Source: three-view drawing plus pictorial views. Frame: mm from the lowest corner of the part. A direction names the side the tool comes from. Coordinates: 2 decimals unless noted, no trailing zeros. Write each loop counter-clockwise with the first axis right and the second up, starting at its lowest first coordinate (ties: lowest second). Pieces come first, ordered by that corner, then holes. Notation, with made-up numbers: (12.5, 25) -> (49.5, 25) arc R20 ccw to (49.5, 47) -> close; hole circle Ø2 at (36, 60). An arc over 180 degrees is marked (long way). One line per question, with ' | ' between items. Start each with the question number.
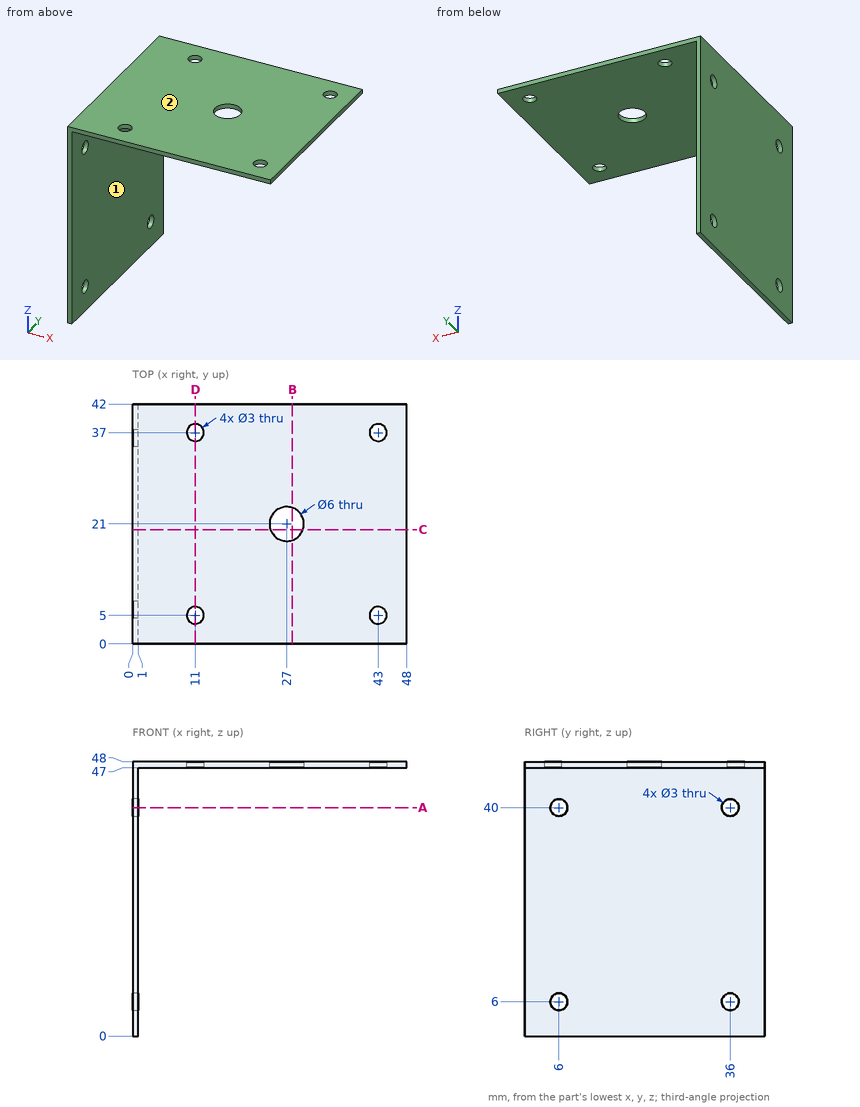
1) Section C-C, the plane y = 20. Return loops of the section in (x, z), then the cut area to 3 significant figures.
2) Section A-A, the plane z = 40. Return loops of the section in (x, y), then the cut area to 3 significant figures.
3) Ray query, line 1 (Y direction, x = 0.3, z = 6); line 2 (Z direction, x = 0.45, y = 36); line 3 (Y direction, x = 11, z = 47.3). Return the intervals inside material, ascending.
4) Section B-B, the plane x = 28. Return loops of the section in (y, z), then the cut area to 3 significant figures.
5) Section D-D, the plane x = 11. Return loops of the section in (y, z), then the cut area to 3 significant figures.
6) Access query for the marked faces 1 and 2. Directions: +Z, -Z, +X, -X, +Y, -Y. A direction counts if a zero-diameter tool reaches every point of the face in a straight line with its end or side. Return the directions, or none.
7) First-contact query: P1, Ø3.5, axis at x = 43, y = 5, coming from the -Z side; P2, Ø3.5, axis at y = 6, z = 6, coming from the +X side. Flat tips, straight axial feed; report the tip coordinate or a pass-through.
Answer block:
1) outline: (0, 0) -> (1, 0) -> (1, 47) -> (24.17, 47) -> (24.17, 48) -> (0, 48) -> close; (29.83, 47) -> (48, 47) -> (48, 48) -> (29.83, 48) -> close | area: 89.3 mm2
2) outline: (0, 0) -> (1, 0) -> (1, 4.5) -> (0, 4.5) -> close; (0, 7.5) -> (1, 7.5) -> (1, 34.5) -> (0, 34.5) -> close; (0, 37.5) -> (1, 37.5) -> (1, 42) -> (0, 42) -> close | area: 36.0 mm2
3) line 1: y = 0 to 4.5, 7.5 to 34.5, 37.5 to 42 | line 2: z = 0 to 4.5, 7.5 to 38.5, 41.5 to 48 | line 3: y = 0 to 3.5, 6.5 to 35.5, 38.5 to 42
4) outline: (0, 47) -> (18.17, 47) -> (18.17, 48) -> (0, 48) -> close; (23.83, 47) -> (42, 47) -> (42, 48) -> (23.83, 48) -> close | area: 36.3 mm2
5) outline: (0, 47) -> (3.5, 47) -> (3.5, 48) -> (0, 48) -> close; (6.5, 47) -> (35.5, 47) -> (35.5, 48) -> (6.5, 48) -> close; (38.5, 47) -> (42, 47) -> (42, 48) -> (38.5, 48) -> close | area: 36.0 mm2
6) face 1: -Z, +X, +Y, -Y | face 2: +Z, +X, -X, +Y, -Y
7) P1: stops at z = 47 | P2: stops at x = 1
